```python
from build123d import *

# Parameters (mm, degrees)
SKETCH1_R           = 7.65
BOSS_EXTRUDE1_DEPTH = 9
FILLET1_R           = 1
SKETCH2_R           = 1.5
SKETCH2_R_2         = 1.435
BOSS_EXTRUDE2_DEPTH = 2.5


with BuildPart() as part:
    # Sketch1 → Boss-Extrude1 (new body)
    with BuildSketch(Plane.XY):
        with BuildLine():
            Line((6.385, 0), (22.385, 0))
            Line((22.385, 0), (28.77, 4))
            Line((28.77, 4), (28.77, 33.652501624))
            ThreePointArc((28.77, 33.652501624), (14.385, 43.38), (0, 33.652501624))
            Line((0, 33.652501624), (0, 4))
            Line((0, 4), (6.385, 0))
        make_face()
        with Locations((14.385, 28.04)):
            Circle(SKETCH1_R, mode=Mode.SUBTRACT)
    extrude(amount=BOSS_EXTRUDE1_DEPTH)

    # Fillet1
    fillet1_edges = [part.edges().sort_by_distance(p)[0] for p in [
        (25.5775, 2, 9),
        (0, 4, 4.5),
        (28.77, 4, 4.5),
        (22.385, 0, 4.5),
        (6.385, 0, 4.5),
        (28.77, 18.826250812, 9),
        (14.385, 43.38, 9),
        (6.735, 28.04, 0),
        (6.735, 28.04, 9),
        (0, 18.826250812, 9),
        (3.1925, 2, 9),
        (14.385, 0, 9),
    ]]
    fillet(fillet1_edges, radius=FILLET1_R)

    # Sketch2 → Boss-Extrude2 (add)
    # profile 1 of 2: a face of its own
    with BuildSketch(Plane(origin=(0, 0, 0), x_dir=(-1, 0, 0), z_dir=(0, 0, -1))):
        with BuildLine():
            Line((-28.77, 33.652501624), (-38.229616207, 30.786722159))
            ThreePointArc((-38.229616207, 30.786722159), (-40.2675, 28.04), (-38.229616207, 25.293277841))
            Line((-38.229616207, 25.293277841), (-28.77, 22.427498376))
            Line((-28.77, 22.427498376), (-28.77, 33.652501624))
        make_face()
        with Locations((-30.6, 28.04)):
            Circle(SKETCH2_R, mode=Mode.SUBTRACT)
        with Locations((-37.3975, 28.04)):
            Circle(SKETCH2_R_2, mode=Mode.SUBTRACT)
    # profile 2 of 2: a face of its own
    with BuildSketch(Plane(origin=(0, 0, 0), x_dir=(-1, 0, 0), z_dir=(0, 0, -1))):
        with BuildLine():
            Line((0, 22.427498376), (9.459616207, 25.293277841))
            ThreePointArc((9.459616207, 25.293277841), (11.4975, 28.04), (9.459616207, 30.786722159))
            Line((9.459616207, 30.786722159), (0, 33.652501624))
            Line((0, 33.652501624), (0, 22.427498376))
        make_face()
        with Locations(Location((8.6275, 28.04, 0), (0, 0, 180))):
            Circle(SKETCH2_R_2, mode=Mode.SUBTRACT)
        with Locations(Location((1.83, 28.04, 0), (0, 0, 180))):
            Circle(SKETCH2_R, mode=Mode.SUBTRACT)
    extrude(amount=-BOSS_EXTRUDE2_DEPTH)


solid = part.part
```
Geometry: final body of the model. Coordinates: model frame, mm. A direction names the side the tool comes from. Coordinates: 2 decimals unless noted, no trailing zeros. Order: outer loops, then holes, each group sorted by start corner. A loop starts at its lowest first (then second) coordinate and runs counter-clockwise, first axis right, second up. Notation, with made-up numbers: (68.25, -18) - (87.25, -18) arc R35 ccw to (87.25, 17) - close; hole circle Ø10 at (32, 78.5). An arc over 180 degrees is marked (long way). Return JSON: item names as keys, results as strings. Group by question number.
1. Pull-direction query (X, two-part tool) for faces 4 (the face through (29.17, 28.49, 1.23)), 5 (the face through (-4, 28, 2.5)), 6 (the face through (25.353, 2.196, 8.699)); classes: pulls with the +X half, pulls with the -X half, needs draft (parallel to the pull), parting line crosses it, or undercut.
2. Cut plane D-D (y = 9.5). Output: boundary loops of the cut face in (x, z), plus the area to 3 significant figures.
3. Cut plane B-B (x = 31.5). Output: boundary loops of the cut face in (y, z), plus the area to 3 significant figures.
4. Pin query (flat end, axial travel): pin 1 (9 mm diameter, centred on x = -8, y = 30.5, fed in from +Z); pin 2 (4 mm diameter, centred on x = 30.6, y = 28.04, fed in from +Z); pin 3 (2 mm diameter, centred on x = 21.5, z = 5, fed in from +Y). Return the tip coordinate at first contact, or that it passes through.
5. Cut plane A-A (y = 28.04). Count the separate pieces of the cut face and the enclosed holes in it, plus the area to 3 significant figures.
6. Set-up query: faces 1 (the face through (33, 28, 2.5)), 2 (the face through (0, 19, 5)), 3 (the face through (28.77, 19, 4)). Return all of +Z, -Z, +X, -X, +Y, -Y with unobstructed straight access to the full face (end or side cutting, diameter ignored); none if empty.
7. Material intervals for line 1 along Z through (x, y) = (-1.5, 23); line 2 along X through (y, z) = (15, 5.5); line 3 along Y through (x, z) = (20, 1.25), sorted ascending. Write a range as [from, to].
Resolved:
{
 "1": {"face 4": "undercut", "face 5": "needs draft", "face 6": "pulls with the +X half"},
 "2": {"outline": "(0, 0) - (28.77, 0) - (28.77, 8) arc R1 ccw to (27.77, 9) - (1, 9) arc R1 ccw to (0, 8) - close", "area": "259 mm²"},
 "3": {"outline": "(23.25, 0) - (26.84, 0) - (26.84, 2.5) - (23.25, 2.5) - close; (29.24, 0) - (32.83, 0) - (32.83, 2.5) - (29.24, 2.5) - close", "area": "17.9 mm²"},
 "4": {"pin 1": "stops at z = 2.5", "pin 2": "stops at z = 8.56", "pin 3": "stops at y = 42.12"},
 "5": {"separate pieces": "6", "enclosed holes": "0", "area": "148 mm²"},
 "6": {"face 1": "+Z, +X, +Y, -Y", "face 2": "+Z, -X, -Y", "face 3": "+Z, +X, -Y"},
 "7": {"line 1": "z = [0, 2.5]", "line 2": "x = [0, 28.77]", "line 3": "y = [0, 22.84], [33.24, 42.33]"}
}
